Could you check a few things on this model? Use its own coordinates, in mm. Face numbers are marked on the shaded views. A direction names the side the tool comes from. Coordinates: 2 decimals unless noted, no trailing zeros. Loops run counter-clockwise (first coordinate to the right, second up) from the corner with the lowest first, then second, coordinate; pieces in that order, holes last. Notation, with made-up numbers: (-18.5, 83.25) - (20.5, 83.25) arc R19 cw to (20.5, 94.25) - close; hole circle Ø8 at (80, 18.25). An arc over 180 degrees is marked (long way). Use CSV: the item, a comma, the result in double quotes.
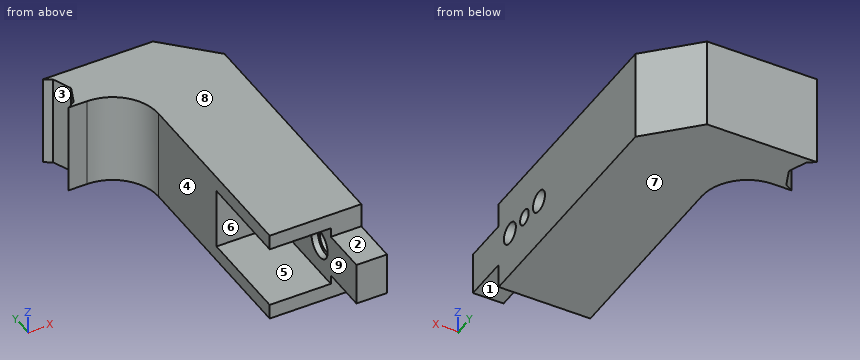
Autodesk Inventor part; units mm, degrees
ref_plane "YZ Plane" through (0, 0, 0) normal (1, 0, 0) x (0, 1, 0)
ref_plane "XZ Plane" through (0, 0, 0) normal (0, 1, 0) x (-1, 0, 0)
ref_plane "XY Plane" through (0, 0, 0) normal (0, 0, 1) x (1, 0, 0)
sketch "Sketch1" plane through (0, 0, 0) normal (0, 0, 1) x (1, 0, 0)
  line L0 (0, 0) -> (25, 0)
  line L1 (25, 0) -> (25, 40)
  line L2 (25, 40) -> (0, 40)
  line L3 (0, 40) -> (0, 0)
  dimension "d1" = 25
  dimension "d2" = 40
  dimension "d3" = 25
extrude "Extrusion1" add sketch "Sketch1" against normal blind 30
sketch "Sketch2" plane through (25, 0, 0) normal (1, 0, 0) x (0, 0, -1)
  line L0 (0, 0) -> (30, 0)
  circle A0 centre (15, 6.56) radius 2.46
extrude "Extrusion2" cut sketch "Sketch2" against normal blind 30
sketch "Sketch3" plane through (0, 0, 0) normal (-1, 0, 0) x (0, 0, 1)
  line L0 (0, 0) -> (-30, 0)
  line L1 (-25.05, 0) -> (-4.95, 0)
  line L2 (-4.95, 0) -> (-4.95, 33.12)
  line L3 (-4.95, 33.12) -> (-25.05, 33.12)
  line L4 (-25.05, 33.12) -> (-25.05, 0)
  dimension "d11" = 20.1
extrude "Extrusion3" cut sketch "Sketch3" against normal blind 20
sketch "Sketch4" plane through (0, 0, 0) normal (0, -1, 0) x (1, 0, 0)
  line L0 (20, -4.95) -> (20, -25.05)
  line L1 (20, -15) -> (25, -15)
  line L2 (25, 0) -> (25, -30)
  line L3 (20, -8.025) -> (25, -8.025)
  line L4 (25, -8.025) -> (25, -21.975)
  line L5 (25, -21.975) -> (20, -21.975)
  line L6 (20, -21.975) -> (20, -8.025)
  line L7 (20, -8.025) -> (25, -21.975) construction
  line L8 (25, -8.025) -> (20, -21.975) construction
  line L9 (25, -12.54) -> (25, -17.46)
  point P0 (0, 0)
  point P1 (22.5, -15)
  dimension "d14" = 13.95
extrude "Extrusion4" add sketch "Sketch4" along normal blind 15
sketch "Sketch5" plane through (20, 0, 0) normal (-1, 0, 0) x (0, 0, 1)
  circle A0 centre (-15, 6.56) radius 2.46
  circle A1 centre (-15, 6.56) radius 4.7025
  circle A2 centre (-15, 6.56) radius 2.46
  circle A3 centre (-15, 6.56) radius 2.46
  point P0 (0, 0)
  dimension "d17" = 9.405
extrude "Extrusion5" cut sketch "Sketch5" against normal blind 2.1
sketch "Sketch6" plane through (25, 0, 0) normal (1, 0, 0) x (0, 0, -1)
  circle A0 centre (15, 6.56) radius 4.7025
  line L0 (15, 6.56) -> (15, 23.56)
  circle A1 centre (15, 23.56) radius 2.46
  point P0 (0, 0)
  dimension "d20" = 17
  dimension "d21" = 4.92
extrude "Extrusion6" cut sketch "Sketch6" against normal blind 10 contours A1
sketch "Sketch7" plane through (20, 0, 0) normal (-1, 0, 0) x (0, 0, 1)
  circle A0 centre (-15, 23.56) radius 2.46
  circle A1 centre (-15, 23.56) radius 4.7025
  point P0 (0, 0)
  dimension "d24" = 9.405
extrude "Extrusion7" cut sketch "Sketch7" against normal blind 2.1
sketch "Sketch9" plane through (25, 0, 0) normal (1, 0, 0) x (0, 0, -1)
  circle A0 centre (15, 6.56) radius 2.46
  circle A1 centre (15, 6.56) radius 2.46
  circle A2 centre (15, 23.56) radius 2.46
  circle A3 centre (15, 23.56) radius 2.46
  line L0 (30, 40) -> (30, 0)
  line L1 (30, 0) -> (30, 40)
  line L2 (30, 40) -> (0, 40)
  line L3 (0, 40) -> (0, 0)
  line L4 (0, 0) -> (8.025, 0)
  line L5 (21.975, 0) -> (21.975, -15)
  line L6 (21.975, -15) -> (8.025, -15)
  line L7 (8.025, -15) -> (8.025, 0)
  line L8 (0, 0) -> (8.025, 0)
  line L9 (21.975, 0) -> (30, 0)
extrude "Extrusion8" add sketch "Sketch9" along normal blind 5
sketch "Sketch10" plane through (0, 40, 0) normal (0, 1, 0) x (1, 0, 0)
  line L0 (0, 30) -> (30, 30)
  line L1 (30, 0) -> (0, 0)
  line L2 (0, 30) -> (30, 30)
  line L3 (30, 30) -> (30, 0)
  line L4 (30, 0) -> (0, 0)
  line L5 (0, 0) -> (0, 30)
extrude "Extrusion9" add sketch "Sketch10" along normal blind 10
sketch "Sketch12" plane through (30, 0, 0) normal (1, 0, 0) x (0, 0, -1)
  circle A0 centre (15, 6.56) radius 2.46
  line L0 (15, 6.56) -> (15, 15.06)
  circle A1 centre (15, 15.06) radius 2.525
  point P0 (0, 0)
  dimension "d31" = 8.5
  dimension "d33" = 5.05
extrude "Extrusion10" cut sketch "Sketch12" against normal blind 30 contours A1
sketch "Sketch14" plane through (0, 0, 0) normal (0, 0, 1) x (1, 0, 0)
  line L0 (30, 50) -> (0, 50)
  line L1 (0, 50) -> (0, 65)
  line L2 (30, 80) -> (15, 95)
  line L3 (-21, 95) -> (15, 95)
  line L4 (30, 0) -> (30, 50)
  line L5 (30, 80) -> (30, 50)
  arc A0 (0, 65) -> (-15, 80) centre (-15, 65) ccw
  line L6 (-15, 80) -> (-21, 80)
  line L7 (-18.5, 93.5) -> (-21, 95)
  line L8 (-18.5, 81.5) -> (-21, 80)
  line L9 (-16, 87.5) -> (-18.5, 81.5)
  line L10 (-16, 87.5) -> (-18.5, 93.5)
  point P0 (0, 0)
  point P1 (0, 80)
  dimension "d47" = 30
  dimension "d54" = 15
  dimension "d70" = 6
  dimension "d72" = 15
extrude "Extrusion12" add sketch "Sketch14" against normal blind 30
sketch "Sketch15" plane through (0, 0, -25.05) normal (-1, 0, 0) x (0, 0, 1)
  line L0 (0, 33.12) -> (20.1, 33.12)
  line L1 (20.1, 33.12) -> (20.1, 0)
  line L2 (0, 33.12) -> (20.1, 33.12)
  line L3 (20.1, 33.12) -> (20.1, 31.1)
  line L4 (20.1, 31.1) -> (0, 31.1)
  line L5 (0, 31.1) -> (0, 33.12)
  point P0 (25.05, 0)
  dimension "d57" = 2.02
extrude "Extrusion13" add sketch "Sketch15" against normal blind 20
sketch "Sketch17" plane through (30, 0, 0) normal (1, 0, 0) x (0, 0, -1)
  circle A0 centre (15, 23.56) radius 2.46
  circle A1 centre (15, 23.56) radius 3.5
  circle A2 centre (15, 6.56) radius 2.46
  circle A3 centre (15, 6.56) radius 3.5
  point P0 (0, 0)
  dimension "d66" = 7
  dimension "d67" = 7
extrude "Extrusion14" cut sketch "Sketch17" against normal blind 10
properties part number "10mm_x_30mm"
(1) Please list where these lines run through material, in increasing order: line 1 (Y direction, x = 25.5, z = -15) (3 decimals); line 2 (Z direction, x = 22, y = 15); line 3 (Y direction, x = 24.5, z = -15) (3 decimals).
Computed:
line 1,"y = -15 to 3.06, 10.06 to 12.535, 17.585 to 20.06, 27.06 to 84.5"
line 2,"z = -30 to -17.52, -12.48 to 0"
line 3,"y = -15 to 3.06, 10.06 to 12.535, 17.585 to 20.06, 27.06 to 85.5"
(2) Suppose I cut it at B-B (y = 15.06). Write out the boundary of the cut face in (x, z) (3 decimals), plus the area to 4 significant figures.
Computed:
outline,"(0, -30) - (30, -30) - (30, -17.525) - (20, -17.525) - (20, -25.05) - (0, -25.05) - close; (0, -4.95) - (20, -4.95) - (20, -12.475) - (30, -12.475) - (30, 0) - (0, 0) - close"
area,"447.5 mm²"
(3) Suppose I cut it at C-C (x = 16). Write out the boundary of the cut face in (y, z).
Computed:
outline,"(0, -30) - (94, -30) - (94, 0) - (0, 0) - (0, -4.95) - (31.1, -4.95) - (31.1, -25.05) - (0, -25.05) - close"
(4) Which directions (+Z, -Z, +X, -X, +Y, -Y) give clear straight access to the entire face, cutting with the end or side of a thin tool? Please do the marked faces 1, 2, 3, 4 and 5.
Computed:
face 1,"-Z, +X, -X, -Y"
face 2,"+Z, +X, -X, -Y"
face 3,"+Z, -Z, -X"
face 4,"+Z, -Z, -X, -Y"
face 5,"-X, -Y"
(5) Thinking about a two-plate mould opening in Z: for the marked faces 6, 7, 8 and 9, which applies, +Z half, -Z half, draft (parallel to the pull), parting line (faces both ways), or undercut?
Computed:
face 6,"undercut"
face 7,"-Z half"
face 8,"+Z half"
face 9,"undercut"
(6) Suppose I cut it at D-D (z = -27). Write out the boundary of the cut face in (x, y).
Computed:
outline,"(-21, 80) - (-15, 80) arc R15 cw to (0, 65) - (0, 0) - (30, 0) - (30, 80) - (15, 95) - (-21, 95) - (-18.5, 93.5) - (-16, 87.5) - (-18.5, 81.5) - close"
(7) Will these pins go through, and if not, where does the flat tip stop? pin 1 (11 mm diameter, centred on x = 24.5, y = -7, fed in from -Z) (3 decimals); pin 2 (1.8 mm diameter, centred on x = -19.5, z = -18.5, fed in from -Y); pin 3 (5 mm diameter, centred on x = 26, y = -6.5, fed in from +Z) (3 decimals).
Computed:
pin 1,"stops at z = -21.975"
pin 2,"stops at y = 80"
pin 3,"stops at z = -8.025"
(8) Suppose I cut it at A-A (z = -15). State how many separate pieces and enclosed holes the cut face has, plus the area to 3 significant figures.
Computed:
separate pieces,"4"
enclosed holes,"0"
area,"2,380 mm²"
